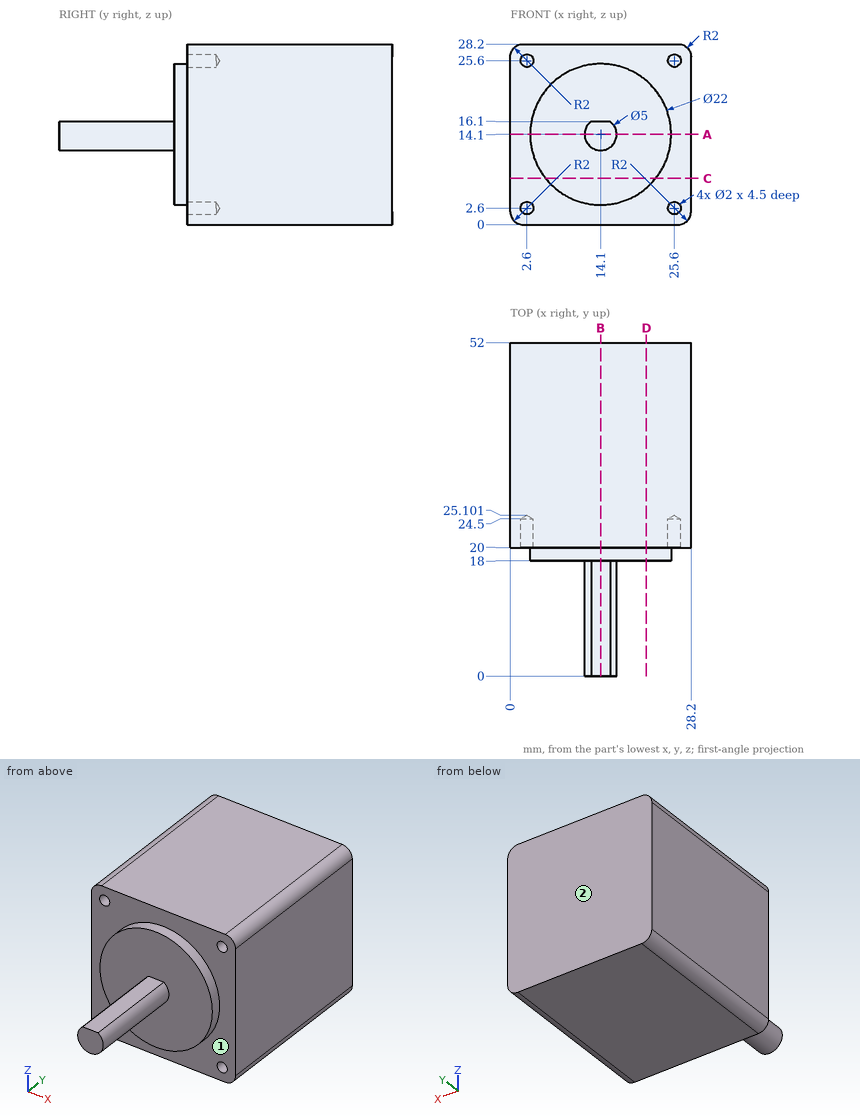
Input: dimensioned drawing with shaded views. Units: mm. Origin: part minimum x, y, z. A direction names the side the tool comes from. Give positions to 0.01 mm unless a question says otherwise; leave off trailing zeros. Loops run counter-clockwise (first coordinate to the right, second up) from the corner with the lowest first, then second, coordinate; pieces in that order, holes last. Notation, with made-up numbers: (-28.5, 22) -> (-15.5, 22) arc R25 ccw to (-15.5, 40) -> close; hole circle Ø10 at (18.5, 32). An arc over 180 degrees is marked (long way). Return JSON: item names as keys, results as strings.
Item 1: Section C-C, the plane z = 7.25. Output: boundary loops of the cut face in (x, y).
Filled in:
{"outline": "(0, 20) -> (5.49, 20) -> (5.49, 18) -> (22.71, 18) -> (22.71, 20) -> (28.2, 20) -> (28.2, 52) -> (0, 52) -> close"}
Item 2: Pin query (flat end, axial travel): P1, Ø4, axis at x = 23.5, y = 14.5, coming from the -Z side; P2, Ø5, axis at x = 16, y = 11.5, coming from the +Z side; P3, Ø3, axis at y = 10, z = 16, coming from the -X side; P4, Ø3, axis at x = 25.6, z = 2.6, coming from the -Y side. Return the tip coordinate at first contact, or that it passes through.
Filled in:
{"P1": "through", "P2": "z = 16.1", "P3": "x = 11.63", "P4": "y = 20"}
Item 3: Line query: line 1 (X direction, y = 23.5, z = 2.6); line 2 (Y direction, x = 13, z = 2). Output: solid intervals per line, ascending.
Filled in:
{"line 1": "0 to 1.6, 3.6 to 24.6, 26.6 to 28.2", "line 2": "20 to 52"}
Item 4: Section D-D, the plane x = 21.25. Output: boundary loops of the cut face in (y, z).
Filled in:
{"outline": "(18, 5.74) -> (20, 5.74) -> (20, 0) -> (52, 0) -> (52, 28.2) -> (20, 28.2) -> (20, 22.46) -> (18, 22.46) -> close"}
Item 5: Section B-B, the plane x = 14.1. Output: boundary loops of the cut face in (y, z).
Filled in:
{"outline": "(0, 11.6) -> (18, 11.6) -> (18, 3.1) -> (20, 3.1) -> (20, 0) -> (52, 0) -> (52, 28.2) -> (20, 28.2) -> (20, 25.1) -> (18, 25.1) -> (18, 16.1) -> (0, 16.1) -> close"}
Item 6: Section A-A, the plane z = 14.1. Output: boundary loops of the cut face in (x, y).
Filled in:
{"outline": "(0, 20) -> (3.1, 20) -> (3.1, 18) -> (11.6, 18) -> (11.6, 0) -> (16.6, 0) -> (16.6, 18) -> (25.1, 18) -> (25.1, 20) -> (28.2, 20) -> (28.2, 52) -> (0, 52) -> close"}
Item 7: Access query for the marked faces 1 and 2. Directions: +Z, -Z, +X, -X, +Y, -Y. A direction counts if a zero-diameter tool reaches every point of the face in a straight line with its end or side. Return the directions, or none.
Filled in:
{"face 1": "-Y", "face 2": "+Z, -Z, +X, -X, +Y"}
